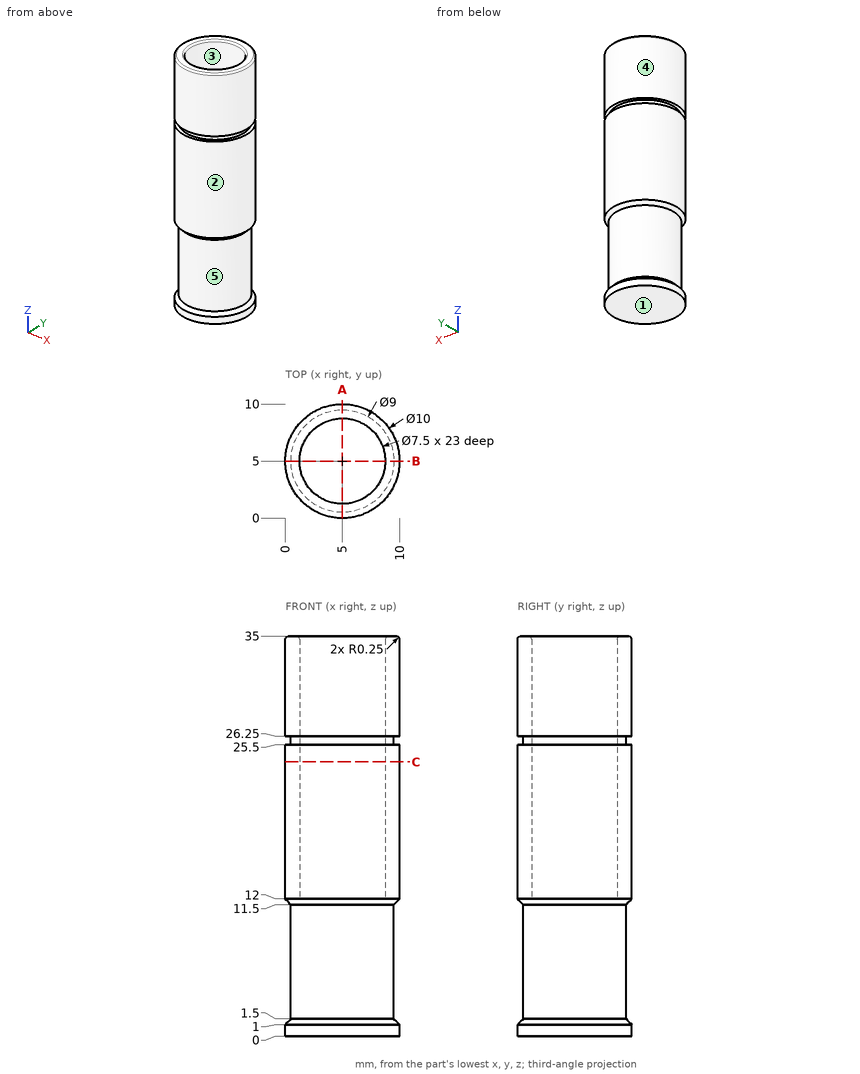
Answer from the drawing. Dimensions are ordinates in mm from the lowest x, y and z of the part. A direction names the side the tool comes from. Give positions to 0.01 mm unless a question says otherwise; leave off trailing zeros. Loops run counter-clockwise (first coordinate to the right, second up) from the corner with the lowest first, then second, coordinate; pieces in that order, holes last.
Item 1: A cutting plane is placed at C-C (z = 24). Give the vertices of the cut face in (x, y).
Derived:
outline: circle Ø10 at (5, 5); hole circle Ø7.5 at (5, 5)
Item 2: Determine the mould class of the marked faces 1, 2 and 3 for opening direction X: +X half, -X half, draft (parallel to the pull), parting line (faces both ways), or undercut.
Derived:
face 1: draft
face 2: parting line
face 3: undercut
Item 3: A tool of negligible diameter and unlimited length cuts with its end or side. For the marked faces 4 and 5, from which of +Z, -Z, +X, -X, +Y, -Y can it reach the whole face along a straight path? Write none if from no direction.
Derived:
face 4: +Z, -Z
face 5: none
Item 4: Find the intervals of material crossed by line 1 along Y through (x, z) = (5, 27.5); line 2 along Z through (x, y) = (6.25, 4.25); line 3 along X through (y, z) = (4.5, 27), in increasing order.
Derived:
line 1: y = 0 to 1.25, 8.75 to 10
line 2: z = 0 to 12
line 3: x = 0.03 to 1.28, 8.72 to 9.97
Item 5: A cutting plane is placed at A-A (x = 5). Give the vertices of the cut face in (y, z).
Derived:
outline: (0, 0) - (10, 0) - (10, 1) - (9.5, 1.5) - (9.5, 11.5) - (10, 12) - (10, 25.5) - (9.5, 25.5) - (9.5, 26.25) - (10, 26.25) - (10, 34.75) arc R0.25 ccw to (9.75, 35) - (9, 35) arc R0.25 ccw to (8.75, 34.75) - (8.75, 12) - (1.25, 12) - (1.25, 34.75) arc R0.25 ccw to (1, 35) - (0.25, 35) arc R0.25 ccw to (0, 34.75) - (0, 26.25) - (0.5, 26.25) - (0.5, 25.5) - (0, 25.5) - (0, 12) - (0.5, 11.5) - (0.5, 1.5) - (0, 1) - close
Item 6: Each of these flat-tipped pins is pushed along its axis until it touches: pin 1 Ø4 at (y, z) = (2.5, 27) entering from +X; pin 2 Ø1.5 at (x, z) = (2, 31) entering from -Y; pin 3 Ø1 at (y, z) = (2, 19) entering from -X. Where does it stop, or does it pass through?
Derived:
pin 1: stops at x = 9.97
pin 2: stops at y = 0.53
pin 3: stops at x = 0.67
